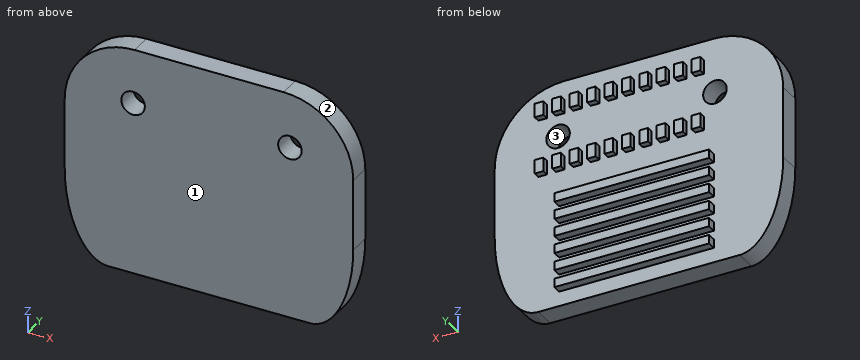
```python
from build123d import *

# Parameters (mm, degrees)
SKETCH8_W                  = 33.098892865
SKETCH8_H                  = 26.166292272
BOSS_EXTRUDE5_DEPTH        = 2.5
M2_5_CLEARANCE_HOLE2_D     = 2.7
M2_5_CLEARANCE_HOLE2_DEPTH = 11.188838164
M2_5_CLEARANCE_HOLE2_TIP   = 0.811161836
SKETCH11_W                 = 1
SKETCH11_H                 = 1.5875
BOSS_EXTRUDE6_DEPTH        = 0.75
LPATTERN1_COUNT            = 10
LPATTERN1_PITCH            = 2
SKETCH11_4_W               = 17.754847744
SKETCH11_4_H               = 1
BOSS_EXTRUDE8_DEPTH        = 1
LPATTERN3_COUNT            = 6
LPATTERN3_PITCH            = 2
FILLET5_R                  = 8
FILLET8_SIZE               = 10
FILLET8_SIZE_2             = 5
FILLET9_SIZE               = 10
FILLET9_SIZE_2             = 5


with BuildPart() as part:
    # Sketch8 → Boss-Extrude5 (new body)
    with BuildSketch(Plane(origin=(0, 0, 0), x_dir=(1, 0, 0), z_dir=(0, 1, 0))):
        with Locations((16.549446433, 13.083146136)):
            Rectangle(SKETCH8_W, SKETCH8_H)
    extrude(amount=-BOSS_EXTRUDE5_DEPTH)

    # M2.5 Clearance Hole2
    with Locations(Plane(origin=(0, 0, 0), x_dir=(1, 0, 0), z_dir=(0, 1, 0))):
        with Locations((7.835608917, 6.278792272), (25.835608917, 6.278792272)):
            Hole(M2_5_CLEARANCE_HOLE2_D / 2, depth=M2_5_CLEARANCE_HOLE2_DEPTH)
            with Locations((0, 0, -(M2_5_CLEARANCE_HOLE2_DEPTH + M2_5_CLEARANCE_HOLE2_TIP / 2))):  # 118° drill point
                Cone(0, M2_5_CLEARANCE_HOLE2_D / 2, M2_5_CLEARANCE_HOLE2_TIP, mode=Mode.SUBTRACT)

    # Sketch11 → Boss-Extrude6 (add)
    with BuildSketch(Plane(origin=(0, 0, 0), x_dir=(1, 0, 0), z_dir=(0, 1, 0))):
        with Locations((27.598892865, 9.572542272)):
            Rectangle(SKETCH11_W, SKETCH11_H)
        with Locations((27.598892865, 2.985042272)):
            Rectangle(SKETCH11_W, SKETCH11_H)
    boss_extrude6 = extrude(amount=BOSS_EXTRUDE6_DEPTH)

    # LPattern1: Boss-Extrude6 ×10
    with Locations(*[(-i * LPATTERN1_PITCH, 0, 0) for i in range(1, LPATTERN1_COUNT)]):
        add(boss_extrude6)

    # Sketch11<4> → Boss-Extrude8 (add)
    with BuildSketch(Plane(origin=(0, 0, 0), x_dir=(1, 0, 0), z_dir=(0, 1, 0))):
        with Locations((16.835608917, 13.981416476)):
            Rectangle(SKETCH11_4_W, SKETCH11_4_H)
    boss_extrude8 = extrude(amount=BOSS_EXTRUDE8_DEPTH)

    # LPattern3: Boss-Extrude8 ×6
    with Locations(*[(0, 0, -i * LPATTERN3_PITCH) for i in range(1, LPATTERN3_COUNT)]):
        add(boss_extrude8)

    # Fillet5
    fillet5_edges = [part.edges().sort_by_distance(p)[0] for p in [
        (33.098892865, -1.25, 0),
        (0, -1.25, 0),
    ]]
    fillet(fillet5_edges, radius=FILLET5_R)

    # Fillet8
    # an asymmetric fillet: 10, 5 mm, written as the material it takes off along each edge
    with BuildSketch(Plane(origin=(33.098892865, 25, -26.166292272), x_dir=(0, 0, 1), z_dir=(0, -1, 0))) as fillet8_piece_1:
        with BuildLine():
            Bezier((FILLET8_SIZE, 0), (0, 0), (0, FILLET8_SIZE_2), weights=[1, 0.707106781, 1])
            Line((0, FILLET8_SIZE_2), (0, 0))
            Line((0, 0), (FILLET8_SIZE, 0))
        make_face()
    extrude(amount=52.5, mode=Mode.SUBTRACT)

    # Fillet9
    # an asymmetric fillet: 10, 5 mm, written as the material it takes off along each edge
    with BuildSketch(Plane(origin=(0, 25, -26.166292272), x_dir=(0, 0, 1), z_dir=(0, -1, 0))) as fillet9_piece_1:
        with BuildLine():
            Bezier((FILLET9_SIZE, 0), (0, 0), (0, -FILLET9_SIZE_2), weights=[1, 0.707106781, 1])
            Line((0, -FILLET9_SIZE_2), (0, 0))
            Line((0, 0), (FILLET9_SIZE, 0))
        make_face()
    extrude(amount=52.5, mode=Mode.SUBTRACT)


solid = part.part
```
The model under review builds one solid part; all positions refer to its coordinate system, in mm. Face numbers are marked on the shaded views. Give positions to 0.01 mm unless a question says otherwise; leave off trailing zeros. Loops run counter-clockwise (first coordinate to the right, second up) from the corner with the lowest first, then second, coordinate; pieces in that order, holes last. Notation, with made-up numbers: (54, -11) - (104, -11) arc R25 ccw to (104, 7) - close; hole circle Ø6 at (-24, -26.75). An arc over 180 degrees is marked (long way). Answer as a JSON object with one key per item and string values.
Q1. Add section A-A on z = -11.25. State the section outline as (x, y) points.
Worked out:
{"outline": "(0, -2.5) - (33.1, -2.5) - (33.1, 0) - (0, 0) - close"}
Q2. Mouldability with a two-part tool opening along Z and no side actions: class the marked faces 1, 2 and 3 as +Z half, -Z half, draft (parallel to the pull), parting line (faces both ways), or undercut.
Worked out:
{"face 1": "draft", "face 2": "+Z half", "face 3": "undercut"}
Q3. Add section B-B on y = -1.85. Count the separate pieces of the cut face and the enclosed holes in it, plus the area to 3 significant figures.
Worked out:
{"separate pieces": "1", "enclosed holes": "2", "area": "806 mm^2"}
Q4. To check wall thickness, follow line 1 along Z through (x, y) = (18, 0.8); line 2 along X through (y, z) = (-0.75, -6.5); line 3 along Z through (x, y) = (27.5, 0.05). State the ranges of each line that lie inside material, in increasing order.
Worked out:
{"line 1": "z = -24.48 to -23.48, -22.48 to -21.48, -20.48 to -19.48, -18.48 to -17.48, -16.48 to -15.48, -14.48 to -13.48", "line 2": "x = 0.14 to 6.5, 9.17 to 24.5, 27.17 to 32.96", "line 3": "z = -10.37 to -8.78, -3.78 to -2.19"}
Q5. Insertion check: pin 1 (0.6 mm diameter, centred on x = 27.5, y = 0.5, fed in from +Z); pin 2 (0.5 mm diameter, centred on y = 0.5, z = -21.5, fed in from -X); pin 3 (2 mm diameter, centred on y = -0.5, z = -5.5, fed in from +X). Each pin has a flat end and moves straight along its axis. Give the tip position at first contact, or say it passes through.
Worked out:
{"pin 1": "stops at z = -2.19", "pin 2": "stops at x = 7.96", "pin 3": "stops at x = 32.96"}
